Source: CAD feature listing. Evaluate the final solid. Frame: model axes, mm. Round coordinates to 2 decimals unless told otherwise and drop trailing zeros. Write each loop counter-clockwise with the first axis right and the second up, starting at its lowest first coordinate (ties: lowest second). Pieces come first, ordered by that corner, then holes. Notation, with made-up numbers: M -34.5,-23 L -1.5,-23 A6 cw -1.5,-16 Z; hole C 62,-30 d8. An arc over 180 degrees is marked long. Answer in a Markdown table with one row per item. Add a question column.
Item 1: Cut plane B-B on x = -31.75. Return loops of the section in (y, z) (1 decimal).
Item 2: Material intervals for probe 1 along X at (y, z) = (3, 0.45) (3 decimals); probe 2 along Y at (x, z) = (-31.75, -1.45) (3 decimals); probe 3 along X at (y, z) = (-0.25, 1.35) (3 decimals), sorted ascending.
Item 3: Mould query, pull axis Y, two halves, no side actions, for faces 1 (the face through (-32.498, -2.374, -1.378)), 2 (the face through (-1, -9.525, 0)), 3 (the face through (-41.275, 0, 0)). Classes: released by +Y, released by -Y, zero draft, split by the parting line, or undercut.
Item 4: Cut plane A-A on y = 0. Return loops of the section in (x, z) (1 decimal).
Item 5: Contact query for flat-ended pins moving along their axis: pin 1 (8 mm diameter, centred on x = 31.75, y = 0, fed in from +Z); pin 2 (5.5 mm diameter, centred on x = -31.75, y = 0, fed in from +Z). Output: stop coordinate, or through.
Item 6: Cut plane C-C on z = -0.1. Return loops of the section in (x, y) (3 decimals), and give its area (3 significant figures).
from build123d import *

# Parameters (mm, degrees)
SKETCH1_W                                    = 82.55
SKETCH1_H                                    = 19.05
EXTRUDE1_DEPTH                               = 1.5875
CSK_FOR_10_FLAT_HEAD_MACHINE_SCREW1_AT_COUNT = 2
CSK_FOR_10_FLAT_HEAD_MACHINE_SCREW1_AT_PITCH = 63.5


with BuildPart() as part:
    # Sketch1 → Extrude1 (new body, symmetric)
    with BuildSketch(Plane.XY):
        Rectangle(SKETCH1_W, SKETCH1_H)
    extrude(amount=EXTRUDE1_DEPTH, both=True)

    # Sketch2 → CSK for #10 Flat Head Machine Screw1 (revolve, cut)
    with BuildSketch(Plane(origin=(-31.75, 0, 1.5875), x_dir=(0, -1, 0), z_dir=(1, 0, 0))):
        Polygon((0, 0), (0, 3.175), (2.4892, 3.175), (2.4892, 2.761229288), (4.8895, 0), align=None)
    csk_for_10_flat_head_machine_screw1 = revolve(axis=Axis((-31.75, 0, 7.9375), (0, 0, -1)), mode=Mode.SUBTRACT)

    # CSK for #10 Flat Head Machine Screw1 at: CSK for #10 Flat Head Machine Screw1 ×2
    with Locations(*[(i * CSK_FOR_10_FLAT_HEAD_MACHINE_SCREW1_AT_PITCH, 0, 0) for i in range(1, CSK_FOR_10_FLAT_HEAD_MACHINE_SCREW1_AT_COUNT)]):
        add(csk_for_10_flat_head_machine_screw1, mode=Mode.SUBTRACT)


solid = part.part
Results below:
| question | item | result |
|---|---|---|
| 1 | outline | M -9.5,-1.6 L -2.5,-1.6 L -2.5,-1.2 L -4.9,1.6 L -9.5,1.6 Z; M 2.5,-1.6 L 9.5,-1.6 L 9.5,1.6 L 4.9,1.6 L 2.5,-1.2 Z |
| 2 | probe 1 | -41.275 to -34.243, -29.257 to 29.257, 34.243 to 41.275 |
| 2 | probe 2 | -9.525 to -2.489, 2.489 to 9.525 |
| 2 | probe 3 | -41.275 to -36.426, -27.074 to 27.074, 36.426 to 41.275 |
| 3 | face 1 | undercut |
| 3 | face 2 | released by -Y |
| 3 | face 3 | zero draft |
| 4 | outline | M -41.3,-1.6 L -34.2,-1.6 L -34.2,-1.2 L -36.6,1.6 L -41.3,1.6 Z; M -29.3,-1.6 L 29.3,-1.6 L 29.3,-1.2 L 26.9,1.6 L -26.9,1.6 L -29.3,-1.2 Z; M 34.2,-1.6 L 41.3,-1.6 L 41.3,1.6 L 36.6,1.6 L 34.2,-1.2 Z |
| 5 | pin 1 | z = 0.56 |
| 5 | pin 2 | z = -0.87 |
| 6 | outline | M -41.275,-9.525 L 41.275,-9.525 L 41.275,9.525 L -41.275,9.525 Z; hole C -31.75,0 d6.845; hole C 31.75,0 d6.845 |
| 6 | area | 1,500 mm2 |
